Source: CAD feature listing. Evaluate the final solid. Frame: model axes, mm. Face numbers are marked on the shaded views. A direction names the side the tool comes from. Give positions to 0.01 mm unless a question says otherwise; leave off trailing zeros. Loops run counter-clockwise (first coordinate to the right, second up) from the corner with the lowest first, then second, coordinate; pieces in that order, holes last. Notation, with made-up numbers: (1, 44) - (60, 44) arc R20 cw to (60, 51) - close; hole circle Ø10 at (30, 23). An arc over 180 degrees is marked (long way). Write each question's results on one line, items separated by ' | '. Start each with the question number.
(1) Cut plane B-B on y = -0.6. Return the cut outline in (x, z), then the cut area to 3 significant figures.
(2) Reachability of the marked faces 1, 2 and 3 from +Z, -Z, +X, -X, +Y, -Y: full face, straight path, thin tool, end or side. Return the list, or none.
(3) Material intervals for line 1 along Z through (x, y) = (-10.5, 0.65); line 2 along X through (y, z) = (0.5, 1.45); line 3 along Y through (x, z) = (-15.5, 1.2) (3 decimals), sorted ascending. Write a range as [from, to].
(4) Cut plane A-A on x = -13. Return the cut outline in (y, z) (3 decimals).
(5) Cut plane C-C on z = -1.75. Return the cut outline in (x, y) (3 decimals), then the cut area to 4 significant figures.
(6) Contact query for flat-ended pins moving along their axis: pin 1 (0.8 mm diameter, centred on x = -15, z = -0.5, fed in from -Y) (3 decimals); pin 2 (1.8 mm diameter, centred on x = -12.5, y = 0, fed in from -Z); pin 3 (0.6 mm diameter, centred on x = -2, y = 1, fed in from +Z). Output: stop coordinate, or through.
from build123d import *

# Parameters (mm, degrees)
SKETCH6_W               = 2.5
SKETCH6_H               = 2.25
BOSS_EXTRUDE1_DEPTH     = 20
CUT_EXTRUDE1_DEPTH      = 21.070578592
CUT_EXTRUDE1_DEPTH_BACK = 21.070578592
SKETCH7_W               = 1
SKETCH7_H               = 0.75
BOSS_EXTRUDE2_DEPTH     = 5


with BuildPart() as part:
    # Sketch6 → Boss-Extrude1 (new, symmetric)
    with BuildSketch(Plane(origin=(0, 0, 0), x_dir=(0, 0, -1), z_dir=(1, 0, 0))):
        Rectangle(SKETCH6_W, SKETCH6_H)
    extrude(amount=BOSS_EXTRUDE1_DEPTH, both=True)

    # Sketch7 → Cut-Extrude1 (cut, two sides: drawn at the far end of the back side and taken through both)
    with BuildSketch(Plane(origin=(0, 0, 0), x_dir=(0, 0, -1), z_dir=(1, 0, 0)).offset(-CUT_EXTRUDE1_DEPTH_BACK)):
        with Locations((0, 0.75)):
            Rectangle(SKETCH7_W, SKETCH7_H)
    extrude(amount=CUT_EXTRUDE1_DEPTH + CUT_EXTRUDE1_DEPTH_BACK, mode=Mode.SUBTRACT)

    # Sketch8 → Boss-Extrude2 (add)
    with BuildSketch(Plane(origin=(0, 0, 0), x_dir=(0, 0, -1), z_dir=(1, 0, 0))):
        Polygon((-2.25, 1.125), (-1.25, 1.125), (-1.25, -1.125), (1.25, -1.125), (1.25, 1.125), (2.25, 1.125), (2.25, -2.125), (-2.25, -2.125), align=None)
    extrude(amount=BOSS_EXTRUDE2_DEPTH)


solid = part.part
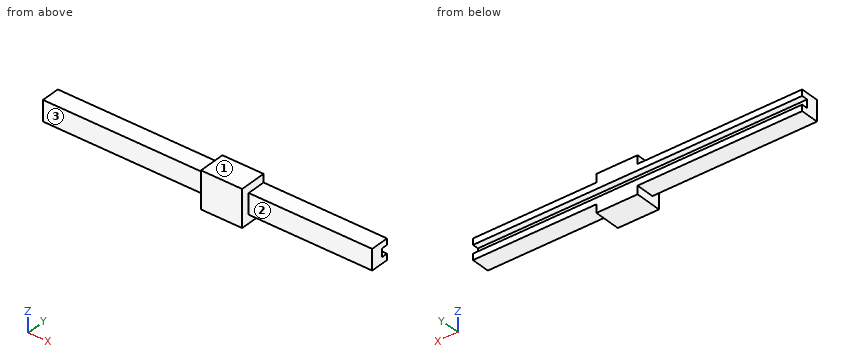
Ans:
1) outline: (-20, -1.25) - (0, -1.25) - (0, -2.25) - (5, -2.25) - (5, -1.25) - (20, -1.25) - (20, 1.25) - (5, 1.25) - (5, 2.25) - (0, 2.25) - (0, 1.25) - (-20, 1.25) - close | area: 110 mm^2
2) face 1: +Z, +X, -X, +Y, -Y | face 2: +Z, -Z, +X, -Y | face 3: +Z, -Z, -X, -Y
3) line 1: [-1.25, -0.5], [0.5, 1.25] | line 2: [0, 5] | line 3: [-1.125, 1.125]
4) outline: (-1.125, -1.25) - (1.125, -1.25) - (1.125, -0.5) - (0.375, -0.5) - (0.375, 0.5) - (1.125, 0.5) - (1.125, 1.25) - (-1.125, 1.25) - close
5) outline: (0, -2.125) - (5, -2.125) - (5, 1.125) - (0, 1.125) - close | area: 16.25 mm^2
6) pin 1: y = -1.125 | pin 2: z = -1.25 | pin 3: z = 1.25
